Source: CAD feature listing. Evaluate the final solid. Frame: model axes, mm. Face numbers are marked on the shaded views. A direction names the side the tool comes from. Give positions to 0.01 mm unless a question says otherwise; leave off trailing zeros. Loops run counter-clockwise (first coordinate to the right, second up) from the corner with the lowest first, then second, coordinate; pieces in that order, holes last. Notation, with made-up numbers: M 35,10 L 49,10 A34 cw 49,41 Z; hole C 54,-28 d11. An arc over 180 degrees is marked long. Put each result on its own line as item: value.
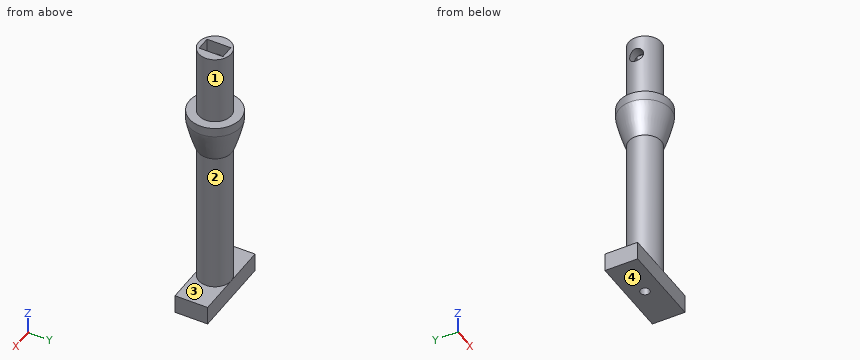
from build123d import *

# Parameters (mm, degrees)
SCHIZZO2_W                    = 18
SCHIZZO2_H                    = 7
ESTRUSIONE_ESTRUSIONE1_DEPTH  = 4
SCHIZZO3_R                    = 3.5
ESTRUSIONE_ESTRUSIONE2_DEPTH  = 55
SCHIZZO4_W                    = 3
SCHIZZO4_H                    = 5.1
TAGLIO_ESTRUSIONE1_DEPTH      = 8.2
TAGLIO_ESTRUSIONE2_REACH      = 62.029
TAGLIO_ESTRUSIONE2_END_RADIUS = 3.5
SCHIZZO5_R                    = 1.5
SCHIZZO6_R                    = 5.5
ESTRUSIONE_ESTRUSIONE3_DEPTH  = 9
RACCORDO1_SIZE                = 2
RACCORDO1_SIZE_2              = 7
SCHIZZO7_R                    = 1
TAGLIO_ESTRUSIONE3_DEPTH      = 2


with BuildPart() as part:
    # Schizzo2 → Estrusione-Estrusione1 (new body)
    with BuildSketch(Plane.XY):
        Rectangle(SCHIZZO2_W, SCHIZZO2_H)
    extrude(amount=ESTRUSIONE_ESTRUSIONE1_DEPTH)

    # Schizzo3 → Estrusione-Estrusione2 (add)
    with BuildSketch(Plane.XY.offset(4)):
        with Locations(Location((0, 0, 0), (0, 0, 270))):
            Circle(SCHIZZO3_R)
    extrude(amount=ESTRUSIONE_ESTRUSIONE2_DEPTH)

    # Schizzo4 → Taglio-Estrusione1 (cut)
    with BuildSketch(Plane.XY.offset(59)):
        Rectangle(SCHIZZO4_W, SCHIZZO4_H)
    extrude(amount=-TAGLIO_ESTRUSIONE1_DEPTH, mode=Mode.SUBTRACT)

    # Taglio-Estrusione2: up to this cylinder (the profile starts inside it)
    taglio_estrusione2_end = Plane(origin=(0, 0, 54.8), z_dir=(0, 0, -1)) * Cylinder(TAGLIO_ESTRUSIONE2_END_RADIUS, 132.058, mode=Mode.PRIVATE)
    # Schizzo5 → Taglio-Estrusione2 (cut, up to the surface)
    with BuildSketch(Plane(origin=(-1.5, 0, 0), x_dir=(0, 0, -1), z_dir=(1, 0, 0)), mode=Mode.PRIVATE) as taglio_estrusione2_sk1:
        with Locations(Location((-54.8, 0, 0), (0, 0, 90))):
            Circle(SCHIZZO5_R)
    taglio_estrusione2_tool1 = extrude(taglio_estrusione2_sk1.sketch, amount=-TAGLIO_ESTRUSIONE2_REACH, mode=Mode.PRIVATE) & taglio_estrusione2_end
    add(taglio_estrusione2_tool1.solids().sort_by_distance((-1.5, 0, 54.8))[0], mode=Mode.SUBTRACT)

    # Schizzo6 → Estrusione-Estrusione3 (add)
    with BuildSketch(Plane.XY.offset(44)):
        Circle(SCHIZZO6_R)
    extrude(amount=-ESTRUSIONE_ESTRUSIONE3_DEPTH)

    # Raccordo1
    # a fillet whose section is not a circle: 7, 2 mm, written as the material it takes off along each edge
    with BuildSketch(Plane(origin=(0, 0, 35), x_dir=(1, 0, 0), z_dir=(0, -1, 0))) as raccordo1_piece_1_section:
        with BuildLine():
            Bezier((5.5 - RACCORDO1_SIZE, 0), (5.5, 0), (5.5, RACCORDO1_SIZE_2), weights=[1, 0.111111111, 1])
            Line((5.5, RACCORDO1_SIZE_2), (5.5, 0))
            Line((5.5, 0), (5.5 - RACCORDO1_SIZE, 0))
        make_face()
    raccordo1_piece_1 = revolve(axis=Axis((0, 0, 35), (0, 0, 1)), mode=Mode.PRIVATE)
    raccordo1_piece_1 = raccordo1_piece_1 - Plane(origin=(0, 0, 35), x_dir=(0, -1, 0), z_dir=(0, 0, -1)) * Cylinder(3.5, 28, mode=Mode.PRIVATE)
    add(raccordo1_piece_1, mode=Mode.SUBTRACT)

    # Schizzo7 → Taglio-Estrusione3 (cut)
    with BuildSketch(Plane(origin=(0, 0, 0), x_dir=(-1, 0, 0), z_dir=(0, 0, -1))):
        Circle(SCHIZZO7_R)
    extrude(amount=-TAGLIO_ESTRUSIONE3_DEPTH, mode=Mode.SUBTRACT)


solid = part.part
1. Draft query along Z for the marked faces 3 and 4. Return one class per face: pulls with the +Z half, pulls with the -Z half, needs draft (parallel to the pull), parting line crosses it, or undercut.
Found:
face 3: undercut
face 4: pulls with the -Z half
2. Material intervals for line 1 (Y direction, x = 0, z = 0.95); line 2 (Z direction, x = -2, y = 0); line 3 (Z direction, x = 7, y = 3.25), sorted ascending. Write a range as from..to.
Found:
line 1: -3.5..-1, 1..3.5
line 2: 0..53.3, 56.3..59
line 3: 0..4
3. Section query A-A (x = 6.5). Output: boundary loops of the cut face in (y, z).
Found:
outline: M -3.5,0 L 3.5,0 L 3.5,4 L -3.5,4 Z
4. Section query B-B (z = 25.5). Output: boundary loops of the cut face in (x, y), plus the area to 3 significant figures.
Found:
outline: C 0,0 d7
area: 38.5 mm^2
5. Section query C-C (z = 54.8). Output: boundary loops of the cut face in (x, y), plus the area to 3 significant figures.
Found:
outline: M -3.16,-1.5 A3.5 ccw long -3.16,1.5 L -1.5,1.5 L -1.5,2.55 L 1.5,2.55 L 1.5,-2.55 L -1.5,-2.55 L -1.5,-1.5 Z
area: 17.5 mm^2
6. Contact query for flat-ended pins moving along their axis: P1, Ø3.5, axis at x = 0, z = 55.5, coming from the -Y side; P2, Ø8, axis at x = -1.5, z = 31, coming from the +Y side; P3, Ø1.6, axis at x = 0, y = 0, coming from the +Z side; P4, Ø3, axis at x = 6.5, z = 7, coming from the +Y side. Output: stop coordinate, or through.
Found:
P1: y = -3.5
P2: y = 3.5
P3: z = 50.8
P4: through
7. Access query for the marked faces 1 and 2. Directions: +Z, -Z, +X, -X, +Y, -Y. A direction counts if a zero-diameter tool reaches every point of the face in a straight line with its end or side. Return the directions, or none.
Found:
face 1: +Z
face 2: none
